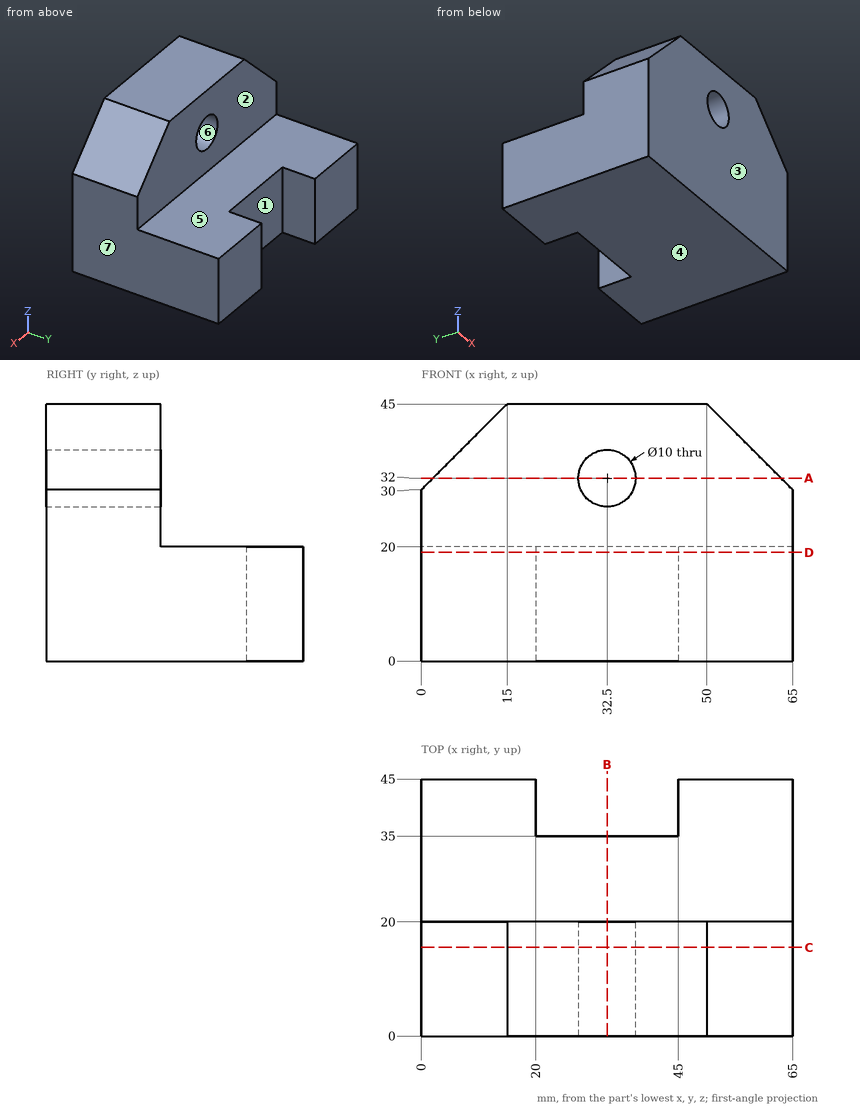
Geometry check sheet. Reference: drawing and pictorial views, mm from the part's lowest x, y, z. A direction names the side the tool comes from. Coordinates: 2 decimals unless noted, no trailing zeros. Order: outer loops, then holes, each group sorted by start corner. A loop starts at its lowest first (then second) coordinate and runs counter-clockwise, first axis right, second up. Notation, with made-up numbers: (-6.75, -12) -> (45.25, -12) arc R25 cw to (45.25, 24) -> close; hole circle Ø10 at (32, -13.75). An arc over 180 degrees is marked (long way). Write item = value, one per line. Start each with the question number.
1) Cross-section at C-C (y = 15.5). Enter the section's corners in (x, z).
2) Access from +Z, -Z, +X, -X, +Y, -Y to the whole of each face (thin tool, end or side, straight path). Record for the marked faces 1, 2 and 3.
3) Cross-section at A-A (z = 32). Enter the section's corners in (x, y), then the cut area to 3 significant figures.
4) Cross-section at B-B (x = 32.5). Enter the section's corners in (y, z), then the cut area to 3 significant figures.
5) Go/stop test with flat-tipped pins: P1, Ø10, axis at x = 34.5, z = 13.5, coming from the +Y side; P2, Ø5, axis at x = 31.5, y = 30, coming from the -Z side; P3, Ø12.5, axis at x = 18, y = 30.5, coming from the +Z side; P4, Ø12.5, axis at x = 33, z = 30, coming from the +Y side. Record where each tip stops, or that it passes through.
6) Material ranges on L1, parallel to X at y = 37.5, z = 5; L2, parallel to Z at x = 32.5, y = 14.75; L3, parallel to Y at x = 14, z = 37.5, recorded low to high.
7) Cross-section at D-D (z = 19). Enter the section's corners in (x, y), then the cut area to 4 significant figures.
8) Mould release check, pull along Z, two halves, no side actions. Record for the marked faces 4, 5, 6 and 7: +Z half, -Z half, draft (parallel to the pull), parting line (faces both ways), or undercut.
Ans:
q1.outline = (0, 0) -> (65, 0) -> (65, 30) -> (50, 45) -> (15, 45) -> (0, 30) -> close; hole circle Ø10 at (32.5, 32)
q2.face_1 = +Z, -Z, +Y
q2.face_2 = +Z, +X, -X, +Y
q2.face_3 = +Z, -Z, +X, -X, -Y
q3.outline = (2, 0) -> (27.5, 0) -> (27.5, 20) -> (2, 20) -> close; (37.5, 0) -> (63, 0) -> (63, 20) -> (37.5, 20) -> close
q3.area = 1,020 mm²
q4.outline = (0, 0) -> (35, 0) -> (35, 20) -> (20, 20) -> (20, 27) -> (0, 27) -> close; (0, 37) -> (20, 37) -> (20, 45) -> (0, 45) -> close
q4.area = 1,000 mm²
q5.P1 = 35
q5.P2 = 0
q5.P3 = 20
q5.P4 = 20
q6.L1 = 0 to 20, 45 to 65
q6.L2 = 0 to 27, 37 to 45
q6.L3 = 0 to 20
q7.outline = (0, 0) -> (65, 0) -> (65, 45) -> (45, 45) -> (45, 35) -> (20, 35) -> (20, 45) -> (0, 45) -> close
q7.area = 2,675 mm²
q8.face_4 = -Z half
q8.face_5 = +Z half
q8.face_6 = undercut
q8.face_7 = draft
